For this review, use the dimensioned drawing (mm, ordinates from the lowest corner) and the shaded views. Give positions to 0.01 mm unless a question says otherwise; leave off trailing zeros. Write each loop counter-clockwise with the first axis right and the second up, starting at its lowest first coordinate (ties: lowest second). Pieces come first, ordered by that corner, then holes. Notation, with made-up numbers: M 18.25,39 L 72.25,39 A11 cw 72.25,58 Z; hole C 80,-25.5 d6. An arc over 180 degrees is marked long. Answer in a Markdown table with one row per item.
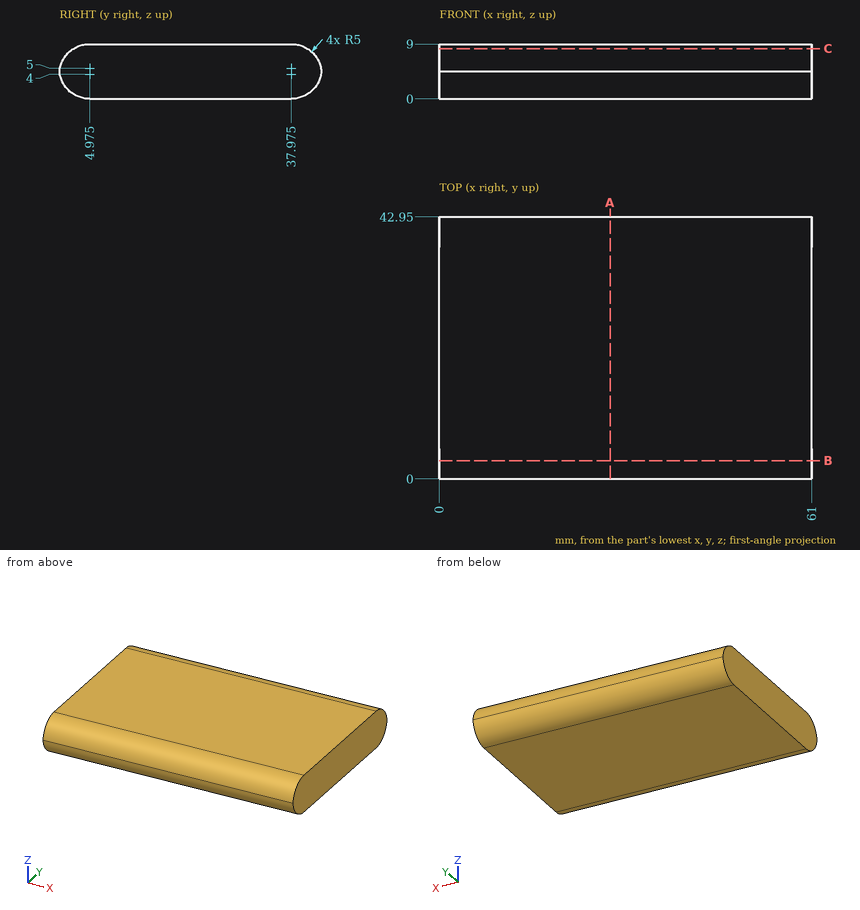
1) Add section A-A (x = 28). Write out the cut boundary in (y, z) (3 decimals).
Geometry says:
| item | result |
|---|---|
| outline | M 0,4.5 A5 ccw 4.975,0 L 37.975,0 A5 ccw 42.95,4.5 A5 ccw 37.975,9 L 4.975,9 A5 ccw Z |
2) To check wall thickness, follow probe 1 along Y at (x, z) = (6, 7.75); probe 2 along Y at (x, z) = (46.5, 6.75); probe 3 along Z at (x, y) = (4.5, 41.5). State the ranges of each line that lie inside material, in increasing order. Write a range as [from, to].
Geometry says:
| item | result |
|---|---|
| probe 1 | [1.67, 41.28] |
| probe 2 | [0.8, 42.15] |
| probe 3 | [1.45, 7.55] |
3) Add section B-B (y = 3). Write out the cut boundary in (x, z).
Geometry says:
| item | result |
|---|---|
| outline | M 0,0.41 L 61,0.41 L 61,8.59 L 0,8.59 Z |
4) Add section C-C (z = 8.25). Write out the cut boundary in (x, y).
Geometry says:
| item | result |
|---|---|
| outline | M 0,2.34 L 61,2.34 L 61,40.61 L 0,40.61 Z |
